```python
from build123d import *

# Parameters (mm, degrees)
SKETCH1_W           = 424
SKETCH1_H           = 295
BOSS_EXTRUDE1_DEPTH = 10


with BuildPart() as part:
    # Sketch1 → Boss-Extrude1 (new body)
    with BuildSketch(Plane(origin=(0, 0, 0), x_dir=(1, 0, 0), z_dir=(0, 1, 0))):
        Rectangle(SKETCH1_W, SKETCH1_H)
        with BuildLine():
            Line((-182, 144.5), (-121, 144.5))
            Line((-121, 144.5), (-121, 83.5))
            ThreePointArc((-121, 83.5), (-111, 73.5), (-121, 63.5))
            Line((-121, 63.5), (-121, 2.5))
            Line((-121, 2.5), (-182, 2.5))
            Line((-182, 2.5), (-182, 144.5))
        make_face(mode=Mode.SUBTRACT)
        with BuildLine():
            Line((-20, 63.5), (-20, 2.5))
            Line((-20, 2.5), (-81, 2.5))
            Line((-81, 2.5), (-81, 144.5))
            Line((-81, 144.5), (-20, 144.5))
            Line((-20, 144.5), (-20, 83.5))
            ThreePointArc((-20, 83.5), (-10, 73.5), (-20, 63.5))
        make_face(mode=Mode.SUBTRACT)
        with BuildLine():
            Line((81, 63.5), (81, 2.5))
            Line((81, 2.5), (20, 2.5))
            Line((20, 2.5), (20, 144.5))
            Line((20, 144.5), (81, 144.5))
            Line((81, 144.5), (81, 83.5))
            ThreePointArc((81, 83.5), (91, 73.5), (81, 63.5))
        make_face(mode=Mode.SUBTRACT)
        with BuildLine():
            Line((182, 63.5), (182, 2.5))
            Line((182, 2.5), (121, 2.5))
            Line((121, 2.5), (121, 144.5))
            Line((121, 144.5), (182, 144.5))
            Line((182, 144.5), (182, 83.5))
            ThreePointArc((182, 83.5), (192, 73.5), (182, 63.5))
        make_face(mode=Mode.SUBTRACT)
        with BuildLine():
            Line((-20, -63.5), (-20, -2.5))
            Line((-20, -2.5), (-81, -2.5))
            Line((-81, -2.5), (-81, -144.5))
            Line((-81, -144.5), (-20, -144.5))
            Line((-20, -144.5), (-20, -83.5))
            ThreePointArc((-20, -83.5), (-10, -73.5), (-20, -63.5))
        make_face(mode=Mode.SUBTRACT)
        with BuildLine():
            Line((-121, -144.5), (-121, -83.5))
            ThreePointArc((-121, -83.5), (-111, -73.5), (-121, -63.5))
            Line((-121, -63.5), (-121, -2.5))
            Line((-121, -2.5), (-182, -2.5))
            Line((-182, -2.5), (-182, -144.5))
            Line((-182, -144.5), (-121, -144.5))
        make_face(mode=Mode.SUBTRACT)
        with BuildLine():
            Line((81, -63.5), (81, -2.5))
            Line((81, -2.5), (20, -2.5))
            Line((20, -2.5), (20, -144.5))
            Line((20, -144.5), (81, -144.5))
            Line((81, -144.5), (81, -83.5))
            ThreePointArc((81, -83.5), (91, -73.5), (81, -63.5))
        make_face(mode=Mode.SUBTRACT)
        with BuildLine():
            Line((182, -63.5), (182, -2.5))
            Line((182, -2.5), (121, -2.5))
            Line((121, -2.5), (121, -144.5))
            Line((121, -144.5), (182, -144.5))
            Line((182, -144.5), (182, -83.5))
            ThreePointArc((182, -83.5), (192, -73.5), (182, -63.5))
        make_face(mode=Mode.SUBTRACT)
    extrude(amount=BOSS_EXTRUDE1_DEPTH)


solid = part.part
```
Check sheet for the modelled part. Datum: model origin and axes. Units: mm. Round coordinates to 2 decimals unless told otherwise and drop trailing zeros. Order: outer loops, then holes, each group sorted by start corner. A loop starts at its lowest first (then second) coordinate and runs counter-clockwise, first axis right, second up. Notation, with made-up numbers: M 0.25,4 L 4.25,4 A9 cw 4.25,10 Z; hole C 30.5,3.25 d11. An arc over 180 degrees is marked long. Answer in a Markdown table with one row per item.
(1) Section check B-B on z = -125. Record the boundary of the cut face in (x, y).
Findings:
| item | result |
|---|---|
| outline | M -212,0 L -182,0 L -182,10 L -212,10 Z; M -121,0 L -81,0 L -81,10 L -121,10 Z; M -20,0 L 20,0 L 20,10 L -20,10 Z; M 81,0 L 121,0 L 121,10 L 81,10 Z; M 182,0 L 212,0 L 212,10 L 182,10 Z |
(2) Section check C-C on z = 73.5. Record the boundary of the cut face in (x, y).
Findings:
| item | result |
|---|---|
| outline | M -212,0 L -182,0 L -182,10 L -212,10 Z; M -111,0 L -81,0 L -81,10 L -111,10 Z; M -10,0 L 20,0 L 20,10 L -10,10 Z; M 91,0 L 121,0 L 121,10 L 91,10 Z; M 192,0 L 212,0 L 212,10 L 192,10 Z |
(3) Material ranges on line 1 along X through (y, z) = (2.5, 106.5); line 2 along Z through (x, y) = (32, 3); line 3 along X through (y, z) = (9.75, -69), recorded low to high. Write a range as from..to.
Findings:
| item | result |
|---|---|
| line 1 | x = -212..-182, -121..-81, -20..20, 81..121, 182..212 |
| line 2 | z = -147.5..-144.5, -2.5..2.5, 144.5..147.5 |
| line 3 | x = -212..-182, -112.07..-81, -11.07..20, 89.93..121, 190.93..212 |
(4) Section check A-A on x = 61. Record the boundary of the cut face in (y, z), plus the area to 3 significant figures.
Findings:
| item | result |
|---|---|
| outline | M 0,-147.5 L 10,-147.5 L 10,-144.5 L 0,-144.5 Z; M 0,-2.5 L 10,-2.5 L 10,2.5 L 0,2.5 Z; M 0,144.5 L 10,144.5 L 10,147.5 L 0,147.5 Z |
| area | 110 mm^2 |
